The model under review builds one solid part; all positions refer to its coordinate system, in mm. Round coordinates to 2 decimals unless told otherwise and drop trailing zeros. Loops run counter-clockwise (first coordinate to the right, second up) from the corner with the lowest first, then second, coordinate; pieces in that order, holes last. Notation, with made-up numbers: (61, 88) -> (91, 88) arc R31 ccw to (91, 114) -> close; hole circle Ø7 at (85, 13). An arc over 180 degrees is marked (long way). Use a Markdown table: item, result. Add a question column.
1) Insertion check: pin 1 (8 mm diameter, centred on x = -31, y = -4.5, fed in from +Z); pin 2 (1.9 mm diameter, centred on x = 67.5, y = -30, fed in from +Z); pin 3 (2 mm diameter, centred on y = 9, z = 7.5, fed in from -X); pin 4 (1 mm diameter, centred on x = 70.5, z = 7.5, fed in from +Y). Each pin has a flat end and moves straight along its axis. Give the tip position at first contact, or say it passes through.
2) Consider section B-B on x = 24. Give the boundary of the cut face in (y, z).
3) Wall thickness on probe 1 along Y at (x, z) = (-67.5, 3.2); probe 2 along X at (y, z) = (-30, 3.65); probe 3 along Y at (x, z) = (-67.5, 0.6): over which ranges is each line inside the solid? List them lowest first.
4) Consider section A-A on y = -9. Give the boundary of the cut face in (x, z).
from build123d import *

# Parameters (mm, degrees)
SKIZZE1_W                                    = 145
SKIZZE1_H                                    = 70
AUFSATZ_LINEAR_AUSTRAGEN1_DEPTH              = 5
VERRUNDUNG1_R                                = 5
FORMSENKUNG_F_R_M3_LINSENSENKSCHRAUB_2_COUNT = 2
FORMSENKUNG_F_R_M3_LINSENSENKSCHRAUB_2_PITCH = 60
FORMSENKUNG_F_R_M3_LINSENSENKSCHRAUB_3_COUNT = 2
FORMSENKUNG_F_R_M3_LINSENSENKSCHRAUB_3_PITCH = 135
FORMSENKUNG_F_R_M3_LINSENSENKSCHRAUB_4_COUNT = 2
FORMSENKUNG_F_R_M3_LINSENSENKSCHRAUB_4_PITCH = 147.732867027
SKIZZE5_W                                    = 5
SKIZZE5_H                                    = 43
AUFSATZ_LINEAR_AUSTRAGEN2_DEPTH              = 4
VERRUNDUNG2_R                                = 0.5
FASE1_SIZE                                   = 0.5
VERRUNDUNG3_R                                = 1.5


with BuildPart() as part:
    # Skizze1 → Aufsatz-Linear austragen1 (new body)
    with BuildSketch(Plane.XY):
        Rectangle(SKIZZE1_W, SKIZZE1_H)
    extrude(amount=AUFSATZ_LINEAR_AUSTRAGEN1_DEPTH)

    # Verrundung1
    verrundung1_edges = [part.edges().sort_by_distance(p)[0] for p in [
        (72.5, -35, 2.5),
        (-72.5, -35, 2.5),
        (-72.5, 35, 2.5),
        (72.5, 35, 2.5),
    ]]
    fillet(verrundung1_edges, radius=VERRUNDUNG1_R)

    # Skizze4 → Formsenkung für M3 Linsensenkschraube mit Schlitz1 (revolve, cut)
    with BuildSketch(Plane(origin=(67.5, 30, 0), x_dir=(0, 1, 0), z_dir=(1, 0, 0))):
        Polygon((0, 0), (0, 5), (1.6, 5), (1.6, 2.55), (3.15, 1), (3.15, 0), align=None)
    formsenkung_f_r_m3_linsensenkschraube_mi = revolve(axis=Axis((67.5, 30, -6.35), (0, 0, 1)), mode=Mode.SUBTRACT)

    # Formsenkung f_r M3 Linsensenkschraub 2: Formsenkung für M3 Linsensenkschraube mit Schlitz1 ×2
    with Locations(*[(0, -i * FORMSENKUNG_F_R_M3_LINSENSENKSCHRAUB_2_PITCH, 0) for i in range(1, FORMSENKUNG_F_R_M3_LINSENSENKSCHRAUB_2_COUNT)]):
        add(formsenkung_f_r_m3_linsensenkschraube_mi, mode=Mode.SUBTRACT)

    # Formsenkung f_r M3 Linsensenkschraub 3: Formsenkung für M3 Linsensenkschraube mit Schlitz1 ×2
    with Locations(*[(-i * FORMSENKUNG_F_R_M3_LINSENSENKSCHRAUB_3_PITCH, 0, 0) for i in range(1, FORMSENKUNG_F_R_M3_LINSENSENKSCHRAUB_3_COUNT)]):
        add(formsenkung_f_r_m3_linsensenkschraube_mi, mode=Mode.SUBTRACT)

    # Formsenkung f_r M3 Linsensenkschraub 4: Formsenkung für M3 Linsensenkschraube mit Schlitz1 ×2
    with Locations(*[Vector(-0.9138115486202572, -0.4061384660534477, 0) * (i * FORMSENKUNG_F_R_M3_LINSENSENKSCHRAUB_4_PITCH) for i in range(1, FORMSENKUNG_F_R_M3_LINSENSENKSCHRAUB_4_COUNT)]):
        add(formsenkung_f_r_m3_linsensenkschraube_mi, mode=Mode.SUBTRACT)

    # Skizze5 → Aufsatz-Linear austragen2 (add)
    with BuildSketch(Plane.XY.offset(5)):
        with Locations((70, 0)):
            Rectangle(SKIZZE5_W, SKIZZE5_H)
    extrude(amount=AUFSATZ_LINEAR_AUSTRAGEN2_DEPTH)

    # Verrundung2
    verrundung2_edges = [part.edges().sort_by_distance(p)[0] for p in [
        (70, 21.5, 9),
        (70, -21.5, 9),
    ]]
    fillet(verrundung2_edges, radius=VERRUNDUNG2_R)

    # Fase1
    fase1_edges = [part.edges().sort_by_distance(p)[0] for p in [
        (72.5, 0, 9),
        (72.5, 21.5, 6.75),
        (72.5, -21.5, 6.75),
        (72.5, 21.353553391, 8.853553391),
        (72.5, -21.353553391, 8.853553391),
    ]]
    chamfer(fase1_edges, length=FASE1_SIZE - 0.0001)  # a hair under: the kernel refuses the full size

    # Verrundung3
    verrundung3_edges = [part.edges().sort_by_distance(p)[0] for p in [
        (72.5, 0, 0),
        (0, -35, 0),
        (-72.5, 0, 0),
        (0, 35, 0),
        (-71.035533906, 33.535533906, 0),
        (71.035533906, 33.535533906, 0),
        (-71.035533906, -33.535533906, 0),
        (71.035533906, -33.535533906, 0),
    ]]
    fillet(verrundung3_edges, radius=VERRUNDUNG3_R)


solid = part.part
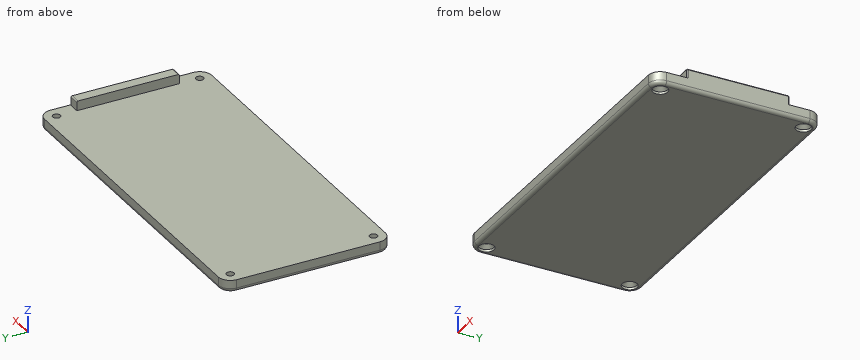
Result set:
| question | item | result |
|---|---|---|
| 1 | pin 1 | z = 5 |
| 1 | pin 2 | through |
| 1 | pin 3 | x = 67.5 |
| 1 | pin 4 | y = 21.5 |
| 2 | outline | (-35, 1.5) arc R1.5 ccw to (-33.5, 0) -> (33.5, 0) arc R1.5 ccw to (35, 1.5) -> (35, 5) -> (-35, 5) -> close |
| 3 | probe 1 | -35 to -31.6, -28.4 to 28.4, 31.6 to 35 |
| 3 | probe 2 | -72.5 to -69.1, -65.9 to 65.9, 69.1 to 72.5 |
| 3 | probe 3 | -34.7 to -33.15, -26.85 to 26.85, 33.15 to 34.7 |
| 4 | outline | (-72.5, 1.5) arc R1.5 ccw to (-71, 0) -> (71, 0) arc R1.5 ccw to (72.5, 1.5) -> (72.5, 8.5) -> (72, 9) -> (67.5, 9) -> (67.5, 5) -> (-72.5, 5) -> close |
